The model under review builds one solid part; all positions refer to its coordinate system, in mm. A direction names the side the tool comes from. Round coordinates to 2 decimals unless told otherwise and drop trailing zeros. Order: outer loops, then holes, each group sorted by start corner. A loop starts at its lowest first (then second) coordinate and runs counter-clockwise, first axis right, second up. Notation, with made-up numbers: M 24.25,35 L 74.25,35 A22 cw 74.25,55 Z; hole C 31.5,26 d2. An arc over 180 degrees is marked long. Use a Markdown table: item, result. Add a question column.
1. The part is to be moulded in two halves that separate along Y. For faces 1 (the cylindrical face through (11.923, 3.755, 0.493)), 2 (the flat face through (1, -1, 11.7)), 3 (the cylindrical face through (7.599, -3.013, 0.493)), say which applies: +Y half, -Y half, draft (parallel to the pull), parting line (faces both ways), or undercut.
2. Insertion check: P1, Ø1.5, axis at y = 8, z = 1, coming from the +X side; P2, Ø4, axis at x = -7.79, y = 4.5, coming from the -Z side; P3, Ø5, axis at x = 5.5, z = 1.5, coming from the -Y side; P4, Ø4, axis at x = -9, y = 1.5, coming from the +Z side. Each pin has a flat end and moves straight along its axis. Give the tip position at first contact, or say it passes through.
3. Consider section C-C on x = -5.5. State the section outline as (y, z) points.
4. Consider section D-D on y = -9. State the section outline as (x, z) points, then the cut area to 3 significant figures.
5. For faces 4 (the cylindrical face through (-3.746, 0.165, 6.275)), 5 (the cylindrical face through (-0.325, -10.464, 0.493)), 6 (the cylindrical face through (-0.596, -2.685, 5.522)), list the 3-axis set-ups (+Z, -Z, +X, -X, +Y, -Y) from which the entire face can be reached by the end or side of a thin tool; tool diameter is ignored.
6. Consider section A-A on y = 0. State the section outline as (x, z) points, then the cut area to 4 significant figures.
7. Consider section B-B on x = 0. Count the separate pieces of the cut face and the enclosed holes in it, then the cut area to 4 significant figures.
8. To check wall thickness, follow probe 1 along Y at (x, z) = (0, 8.25); probe 2 along Y at (x, z) = (0, 0.55); probe 3 along Z at (x, y) = (-5, -8.75). State the ranges of each line that lie inside material, in increasing order.
from build123d import *

# Parameters (mm, degrees)
SKETCH_1_R      = 12.5
SKETCH_1_R_2    = 2.75
SKETCH_1_R_3    = 1.5
SKETCH_1_R_4    = 1
EXTRUDE_1_DEPTH = 1
SKETCH_2_R      = 3.75
SKETCH_2_R_2    = 2.75
EXTRUDE_2_DEPTH = 10.2
SKETCH_3_R      = 3.75
SKETCH_3_R_2    = 1
EXTRUDE_3_DEPTH = 0.5


with BuildPart() as part:
    # Эскиз1 → Бобышка-Вытянуть1 (new body)
    with BuildSketch(Plane.XY):
        Circle(SKETCH_1_R)
        Circle(SKETCH_1_R_2, mode=Mode.SUBTRACT)
        with Locations((0, 9)):
            Circle(SKETCH_1_R_3, mode=Mode.SUBTRACT)
        with Locations((7.794228634, 4.5)):
            Circle(SKETCH_1_R_3, mode=Mode.SUBTRACT)
        with Locations((7.794228634, -4.5)):
            Circle(SKETCH_1_R_3, mode=Mode.SUBTRACT)
        with Locations((0, -9)):
            Circle(SKETCH_1_R_3, mode=Mode.SUBTRACT)
        with Locations((-7.794228634, -4.5)):
            Circle(SKETCH_1_R_3, mode=Mode.SUBTRACT)
        with Locations((-7.794228634, 4.5)):
            Circle(SKETCH_1_R_3, mode=Mode.SUBTRACT)
        with Locations((-5.5, 0)):
            Circle(SKETCH_1_R_3, mode=Mode.SUBTRACT)
        with Locations(Location((5.5, 0, 0), (0, 0, 180))):
            Circle(SKETCH_1_R_3, mode=Mode.SUBTRACT)
        with Locations((0, 5.5)):
            Circle(SKETCH_1_R_4, mode=Mode.SUBTRACT)
        with Locations(Location((0, -5.5, 0), (0, 0, 180))):
            Circle(SKETCH_1_R_4, mode=Mode.SUBTRACT)
    extrude(amount=EXTRUDE_1_DEPTH)

    # Эскиз2 → Бобышка-Вытянуть2 (add)
    with BuildSketch(Plane.XY.offset(1)):
        Circle(SKETCH_2_R)
        Circle(SKETCH_2_R_2, mode=Mode.SUBTRACT)
    extrude(amount=EXTRUDE_2_DEPTH)

    # Эскиз3 → Бобышка-Вытянуть3 (add)
    with BuildSketch(Plane.XY.offset(11.2)):
        Circle(SKETCH_3_R)
        Circle(SKETCH_3_R_2, mode=Mode.SUBTRACT)
    extrude(amount=EXTRUDE_3_DEPTH)


solid = part.part
Answer block:
| question | item | result |
|---|---|---|
| 1 | face 1 | parting line |
| 1 | face 2 | draft |
| 1 | face 3 | undercut |
| 2 | P1 | x = 10.18 |
| 2 | P2 | z = 0 |
| 2 | P3 | y = -12.12 |
| 2 | P4 | z = 1 |
| 3 | outline | M -11.22,0 L -1.5,0 L -1.5,1 L -11.22,1 Z; M 1.5,0 L 11.22,0 L 11.22,1 L 1.5,1 Z |
| 4 | outline | M -8.67,0 L -1.5,0 L -1.5,1 L -8.67,1 Z; M 1.5,0 L 8.67,0 L 8.67,1 L 1.5,1 Z |
| 4 | area | 14.3 mm^2 |
| 5 | face 4 | +Z |
| 5 | face 5 | +Z, -Z |
| 5 | face 6 | -Z |
| 6 | outline | M -12.5,0 L -7,0 L -7,1 L -12.5,1 Z; M -4,0 L -2.75,0 L -2.75,11.2 L -1,11.2 L -1,11.7 L -3.75,11.7 L -3.75,1 L -4,1 Z; M 1,11.2 L 2.75,11.2 L 2.75,0 L 4,0 L 4,1 L 3.75,1 L 3.75,11.7 L 1,11.7 Z; M 7,0 L 12.5,0 L 12.5,1 L 7,1 Z |
| 6 | area | 36.65 mm^2 |
| 7 | separate pieces | 6 |
| 7 | enclosed holes | 0 |
| 7 | area | 32.65 mm^2 |
| 8 | probe 1 | -3.75 to -2.75, 2.75 to 3.75 |
| 8 | probe 2 | -12.5 to -10.5, -7.5 to -6.5, -4.5 to -2.75, 2.75 to 4.5, 6.5 to 7.5, 10.5 to 12.5 |
| 8 | probe 3 | 0 to 1 |
